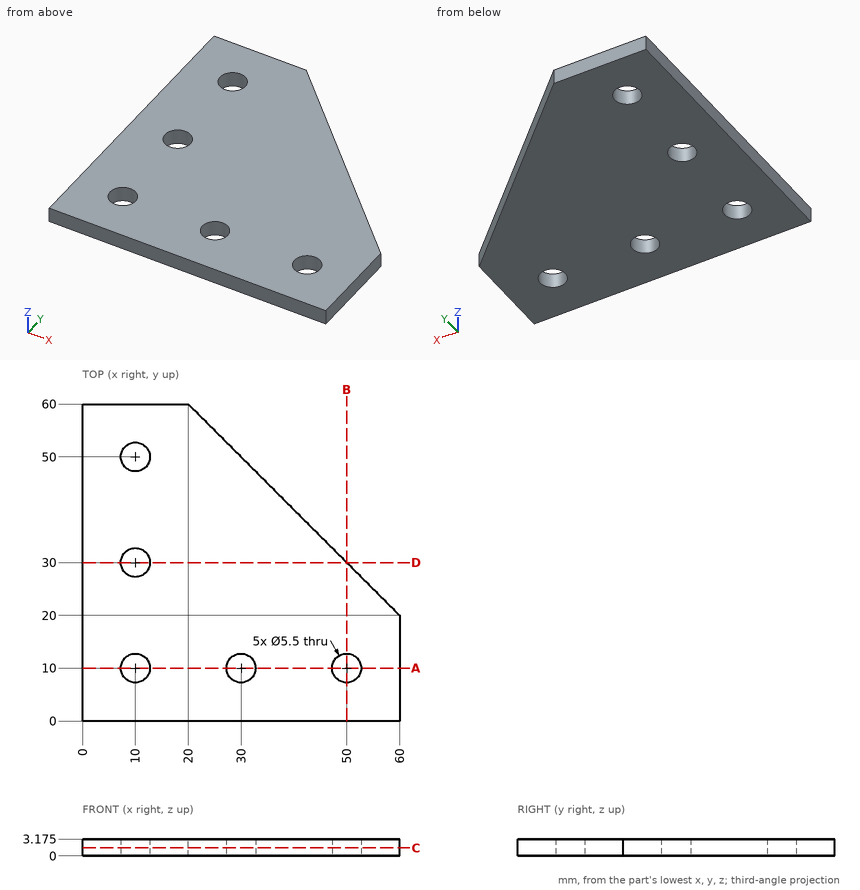
Input: dimensioned drawing with shaded views. Units: mm. Origin: part minimum x, y, z. Give positions to 0.01 mm unless a question says otherwise; leave off trailing zeros. Write each loop counter-clockwise with the first axis right and the second up, starting at its lowest first coordinate (ties: lowest second). Pieces come first, ordered by that corner, then holes.
Q1. Material intervals for probe 1 along Y at (x, z) = (10, 2.5); probe 2 along Y at (x, z) = (11.5, 1.5); probe 3 along Y at (x, z) = (50, 1.35), sorted ascending.
Q2. Section D-D, the plane y = 30. Output: boundary loops of the cut face in (x, z) (3 decimals).
Q3. Section B-B, the plane x = 50. Output: boundary loops of the cut face in (y, z) (3 decimals), plus the area to 3 significant figures.
Q4. Section A-A, the plane y = 10. Output: boundary loops of the cut face in (x, z) (3 decimals).
Q5. Section C-C, the plane z = 1.5. Output: boundary loops of the cut face in (x, y), plus the area to 3 significant figures.
Filled in:
1. probe 1: y = 0 to 7.25, 12.75 to 27.25, 32.75 to 47.25, 52.75 to 60
1. probe 2: y = 0 to 7.7, 12.3 to 27.7, 32.3 to 47.7, 52.3 to 60
1. probe 3: y = 0 to 7.25, 12.75 to 30
2. outline: (0, 0) - (7.25, 0) - (7.25, 3.175) - (0, 3.175) - close; (12.75, 0) - (50, 0) - (50, 3.175) - (12.75, 3.175) - close
3. outline: (0, 0) - (7.25, 0) - (7.25, 3.175) - (0, 3.175) - close; (12.75, 0) - (30, 0) - (30, 3.175) - (12.75, 3.175) - close
3. area: 77.8 mm2
4. outline: (0, 0) - (7.25, 0) - (7.25, 3.175) - (0, 3.175) - close; (12.75, 0) - (27.25, 0) - (27.25, 3.175) - (12.75, 3.175) - close; (32.75, 0) - (47.25, 0) - (47.25, 3.175) - (32.75, 3.175) - close; (52.75, 0) - (60, 0) - (60, 3.175) - (52.75, 3.175) - close
5. outline: (0, 0) - (60, 0) - (60, 20) - (20, 60) - (0, 60) - close; hole circle Ø5.5 at (10, 10); hole circle Ø5.5 at (10, 30); hole circle Ø5.5 at (10, 50); hole circle Ø5.5 at (30, 10); hole circle Ø5.5 at (50, 10)
5. area: 2,680 mm2
